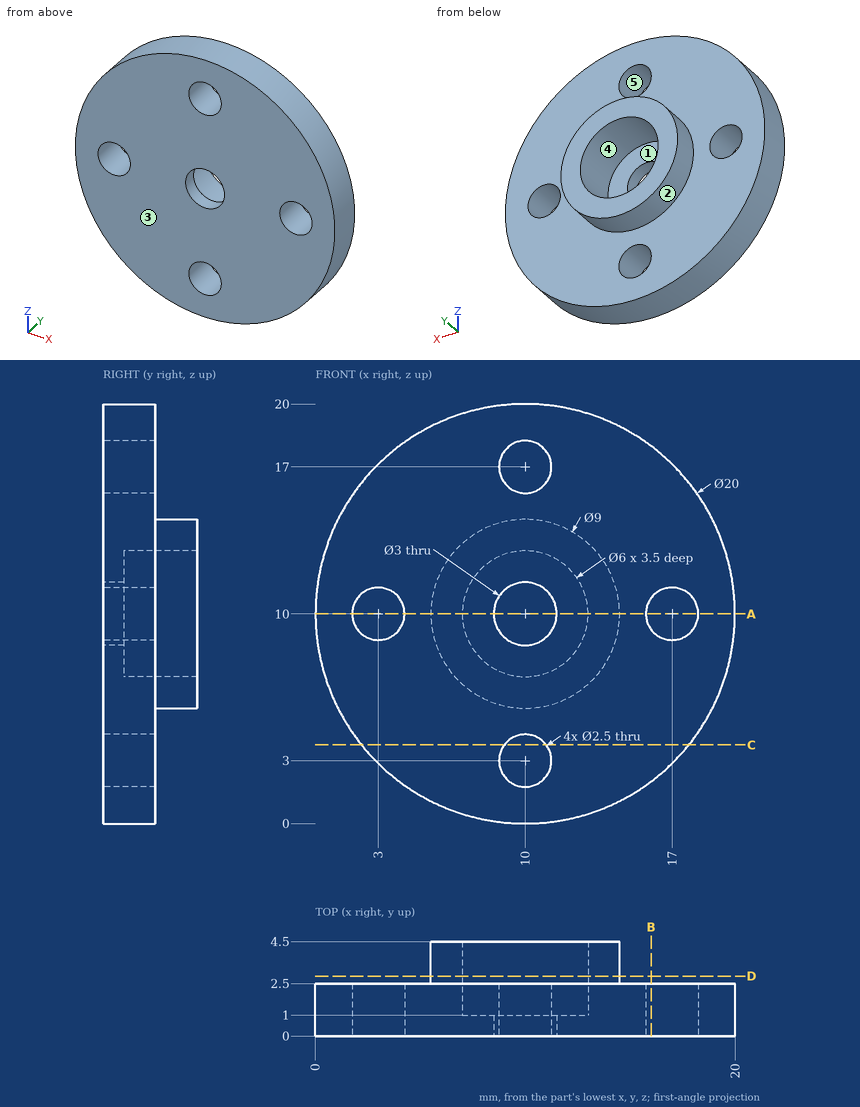
The figure shows three views and two pictorial views of one solid part (mm, origin at its lowest corner). Answer the questions. A direction names the side the tool comes from. Round coordinates to 2 decimals unless told otherwise and drop trailing zeros. Loops run counter-clockwise (first coordinate to the right, second up) from the corner with the lowest first, then second, coordinate; pieces in that order, holes last. Notation, with made-up numbers: M 45.25,-32 L 103.25,-32 A19 ccw 103.25,-1 Z; hole C 57.25,-24 d3. An arc over 180 degrees is marked long. Return JSON: item names as keys, results as strings.
Q1. Find the intervals of material crossed by line 1 along X through (y, z) = (0.4, 10); line 2 along Z through (x, y) = (3, 1.7); line 3 along Z through (x, y) = (10, 2.65), in increasing order. Write a range as from..to.
Results list:
{"line 1": "x = 0..1.75, 4.25..8.5, 11.5..15.75, 18.25..20", "line 2": "z = 2.86..8.75, 11.25..17.14", "line 3": "z = 5.5..7, 13..14.5"}
Q2. Find section C-C, the plane z = 3.75. Determine the outline of the cut face in (x, y).
Results list:
{"outline": "M 2.19,0 L 9,0 L 9,2.5 L 2.19,2.5 Z; M 11,0 L 17.81,0 L 17.81,2.5 L 11,2.5 Z"}
Q3. Which of the six approach directions +Z, -Z, +X, -X, +Y, -Y give full straight-line access (tool end or side, diameter ignored) to the marked faces 4 and 5?
Results list:
{"face 4": "+Y", "face 5": "+Y, -Y"}
Q4. Find section D-D, the plane y = 2.85. Determine the outline of the cut face in (x, z).
Results list:
{"outline": "C 10,10 d9; hole C 10,10 d6"}
Q5. The mould has two halves that part along Z. Classify the marked faces 1, 2 and 3: released by +Z, released by -Z, zero draft, split by the parting line, or undercut.
Results list:
{"face 1": "undercut", "face 2": "split by the parting line", "face 3": "zero draft"}
Q6. Each of these flat-tipped pins is pushed along its axis until it touches: pin 1 Ø1.5 at (x, y) = (16, 2) entering from -Z; pin 2 Ø1.5 at (x, z) = (11, 9.5) entering from +Y; pin 3 Ø2 at (x, z) = (10, 3) entering from -Y; pin 4 Ø2 at (x, y) = (5.5, 2.5) entering from +Z. Where does it stop, or does it pass through?
Results list:
{"pin 1": "stops at z = 1.49", "pin 2": "stops at y = 1", "pin 3": "passes through", "pin 4": "stops at z = 19.37"}
Q7. Find section A-A, the plane z = 10. Determine the outline of the cut face in (x, y).
Results list:
{"outline": "M 0,0 L 1.75,0 L 1.75,2.5 L 0,2.5 Z; M 4.25,0 L 8.5,0 L 8.5,1 L 7,1 L 7,4.5 L 5.5,4.5 L 5.5,2.5 L 4.25,2.5 Z; M 11.5,0 L 15.75,0 L 15.75,2.5 L 14.5,2.5 L 14.5,4.5 L 13,4.5 L 13,1 L 11.5,1 Z; M 18.25,0 L 20,0 L 20,2.5 L 18.25,2.5 Z"}
Q8. Find section B-B, the plane x = 16. Determine the outline of the cut face in (y, z), plus the area to 4 significant figures.
Results list:
{"outline": "M 0,2 L 2.5,2 L 2.5,9.25 L 0,9.25 Z; M 0,10.75 L 2.5,10.75 L 2.5,18 L 0,18 Z", "area": "36.25 mm2"}
